from build123d import *

# Parameters (mm, degrees)
SKETCH1_W                             = 196.85
SKETCH1_H                             = 203.2
BOSS_EXTRUDE1_DEPTH                   = 0.7747
CUT_EXTRUDE7_DEPTH                    = 1.7747
SKETCH4_W                             = 196.85
SKETCH4_H                             = 0.6096
BOSS_EXTRUDE2_DEPTH                   = 12
SKETCH14_W                            = 196.85
SKETCH14_H                            = 11.938
BOSS_EXTRUDE3_DEPTH                   = 0.7747
SKETCH13_W                            = 196.85
SKETCH13_H                            = 0.6096
CUT_EXTRUDE9_DEPTH                    = 12
CSK_FOR_M3_FLAT_HEAD_MACHINE_SCREW3_D = 3.81
SKETCH19_W                            = 182.676330849
SKETCH19_H                            = 33.741187375
BOSS_EXTRUDE4_DEPTH                   = 0.7747
SKETCH21_W                            = 22.718000829
SKETCH21_H                            = 22.312299049
SKETCH21_W_2                          = 21.538835619
SKETCH21_H_2                          = 16.643270878
BOSS_EXTRUDE5_DEPTH                   = 0.7747
SKETCH22_W                            = 13.90531837
SKETCH22_H                            = 14.215216999
SKETCH22_W_2                          = 12.509578485
SKETCH22_H_2                          = 9.075576548
BOSS_EXTRUDE6_DEPTH                   = 0.7747


with BuildPart() as part:
    # Sketch1 → Boss-Extrude1 (new body)
    with BuildSketch(Plane(origin=(0, 0, 0), x_dir=(1, 0, 0), z_dir=(0, 0, -1))):
        with Locations((-104.775, 135.4)):
            Rectangle(SKETCH1_W, SKETCH1_H)
    extrude(amount=BOSS_EXTRUDE1_DEPTH)

    # Sketch2 → Cut-Extrude7 (cut, through all)
    with BuildSketch(Plane(origin=(0, 0, -0.7747), x_dir=(1, 0, 0), z_dir=(0, 0, -1))):
        with BuildLine():
            Line((-135.221253236, 173.5), (-135.221253236, 148))
            ThreePointArc((-135.221253236, 148), (-141.721253236, 141.5), (-148.221253236, 148))
            Line((-148.221253236, 148), (-148.221253236, 173.5))
            ThreePointArc((-148.221253236, 173.5), (-141.721253236, 180), (-135.221253236, 173.5))
        make_face()
        with BuildLine():
            Line((-62.069253236, 173.5), (-62.069253236, 148))
            ThreePointArc((-62.069253236, 148), (-68.569253236, 141.5), (-75.069253236, 148))
            Line((-75.069253236, 148), (-75.069253236, 173.5))
            ThreePointArc((-75.069253236, 173.5), (-68.569253236, 180), (-62.069253236, 173.5))
        make_face()
    extrude(amount=-CUT_EXTRUDE7_DEPTH, mode=Mode.SUBTRACT)

    # Sketch4 → Boss-Extrude2 (add)
    with BuildSketch(Plane.XY):
        with Locations((-104.775, -34.1048)):
            Rectangle(SKETCH4_W, SKETCH4_H)
    extrude(amount=BOSS_EXTRUDE2_DEPTH)

    # Sketch14 → Boss-Extrude3 (add)
    with BuildSketch(Plane.XY):
        with Locations((-104.775, -53.935004147)):
            Rectangle(SKETCH14_W, SKETCH14_H)
    extrude(amount=-BOSS_EXTRUDE3_DEPTH)

    # Sketch13 → Cut-Extrude9 (cut)
    with BuildSketch(Plane.XY.offset(12)):
        with Locations((-104.775, -34.1048)):
            Rectangle(SKETCH13_W, SKETCH13_H)
    extrude(amount=-CUT_EXTRUDE9_DEPTH, mode=Mode.SUBTRACT)

    # CSK for M3 Flat Head Machine Screw3 (through all)
    with Locations(Plane.XY):
        with Locations((-188.645, -72), (-188.645, -222), (-188.645, -197), (-188.645, -172), (-188.645, -147), (-188.645, -122), (-188.645, -97)):
            csk_for_m3_flat_head_machine_screw3 = Hole(CSK_FOR_M3_FLAT_HEAD_MACHINE_SCREW3_D / 2)

    # Mirror1: CSK for M3 Flat Head Machine Screw3 across plane
    add(csk_for_m3_flat_head_machine_screw3.mirror(Plane(origin=(-104.775, 0, 0), x_dir=(0, 0, 1), z_dir=(1, 0, 0))), mode=Mode.SUBTRACT)

    # Sketch19 → Boss-Extrude4 (add)
    with BuildSketch(Plane(origin=(0, 0, -0.7747), x_dir=(-1, 0, 0), z_dir=(0, 0, -1))):
        with Locations((101.266706015, -109.837466763)):
            Rectangle(SKETCH19_W, SKETCH19_H)
    extrude(amount=-BOSS_EXTRUDE4_DEPTH)

    # Sketch21 → Boss-Extrude5 (add)
    with BuildSketch(Plane(origin=(0, 0, -0.7747), x_dir=(-1, 0, 0), z_dir=(0, 0, -1))):
        with Locations((185.571692861, -170.919383368)):
            Rectangle(SKETCH21_W, SKETCH21_H)
        with Locations((24.271371833, -173.753897453)):
            Rectangle(SKETCH21_W_2, SKETCH21_H_2)
    extrude(amount=-BOSS_EXTRUDE5_DEPTH)

    # Sketch22 → Boss-Extrude6 (add)
    with BuildSketch(Plane.XY):
        with Locations((-189.313880795, -220.883843828)):
            Rectangle(SKETCH22_W, SKETCH22_H)
        with Locations((-23.670028487, -197.876391374)):
            Rectangle(SKETCH22_W_2, SKETCH22_H_2)
    extrude(amount=-BOSS_EXTRUDE6_DEPTH)


solid = part.part
Input: part model. Units: mm. Frame: model coordinates. A direction names the side the tool comes from. Round coordinates to 2 decimals unless told otherwise and drop trailing zeros. Order: outer loops, then holes, each group sorted by start corner. A loop starts at its lowest first (then second) coordinate and runs counter-clockwise, first axis right, second up. Notation, with made-up numbers: (46, 8) - (70, 8) arc R23 ccw to (70, 17) - close; hole circle Ø2 at (8, 78.5). An arc over 180 degrees is marked (long way). Answer as a JSON object with one key per item and string values. Group by question number.
(1) Material intervals for probe 1 along X at (y, z) = (-157.5, -0.45); probe 2 along X at (y, z) = (-222, -0.45); probe 3 along Y at (x, z) = (-22, -0.35), sorted ascending. Write a range as from..to.
(2) Draft query along Y for faces 1 (the face through (-106, -137, -0.775)), 2 (the face through (-141.6, -141.5, -0.4)). Return one class per face: released by +Y, released by -Y, zero draft, split by the parting line, or undercut.
(3) Pin query (flat end, axial travel): P1, Ø2.5, axis at x = -188.645, y = -147, coming from the +Z side; P2, Ø4.5, axis at x = -20.905, y = -72, coming from the +Z side. Return the tip coordinate at first contact, or that it passes through.
(4) Cut plane A-A (y = -163.5). Return loops of the section in (x, z).
(5) Cut plane C-C (x = -72.5). Return loops of the section in (y, z).
(6) Reachability of faces 3 (the face through (-106, -137, 0)), 4 (the face through (-68.43, -141.5, -0.39)) from +Z, -Z, +X, -X, +Y, -Y: full face, straight path, thin tool, end or side. Return the list, or none.
(7) Cut plane B-B (z = -0.5). Count the separate pieces of the cut face and the enclosed holes in it, then the cut area to 3 significant figures.
Here are the results:
{
 "1": {"probe 1": "x = -203.2..-148.22, -135.22..-75.07, -62.07..-6.35", "probe 2": "x = -203.2..-22.81, -19..-6.35", "probe 3": "y = -237..-223.56, -220.44..-148.56, -145.44..-73.56, -70.44..-33.8"},
 "2": {"face 1": "zero draft", "face 2": "undercut"},
 "3": {"P1": "passes through", "P2": "stops at z = 0"},
 "4": {"outline": "(-203.2, -0.77) - (-148.22, -0.77) - (-148.22, 0) - (-203.2, 0) - close; (-135.22, -0.77) - (-75.07, -0.77) - (-75.07, 0) - (-135.22, 0) - close; (-62.07, -0.77) - (-6.35, -0.77) - (-6.35, 0) - (-62.07, 0) - close"},
 "5": {"outline": "(-237, -0.77) - (-178.68, -0.77) - (-178.68, 0) - (-237, 0) - close; (-142.82, -0.77) - (-33.8, -0.77) - (-33.8, 0) - (-142.82, 0) - close"},
 "6": {"face 3": "+Z, +X, -X, +Y, -Y", "face 4": "+Z, -Z"},
 "7": {"separate pieces": "1", "enclosed holes": "8", "area": "39,000 mm^2"}
}
